Verification items for the finished model (mm, model axes). A direction names the side the tool comes from. Round coordinates to 2 decimals unless told otherwise and drop trailing zeros. Write each loop counter-clockwise with the first axis right and the second up, starting at its lowest first coordinate (ties: lowest second). Pieces come first, ordered by that corner, then holes. Notation, with made-up numbers: M -16,57.25 L -10,57.25 A20 cw -10,65.25 Z; hole C 63.5,-26 d8. An arc over 180 degrees is marked long. Use a Markdown table: item, result. Add a question column.
from build123d import *

# Parameters (mm, degrees)
FILLET_1_R      = 5
FILLET_2_R      = 10
SKETCH_2_R      = 45
SKETCH_2_R_2    = 35
EXTRUDE_1_DEPTH = 32
SKETCH_3_R      = 35
EXTRUDE_2_DEPTH = 66
SKETCH_4_R      = 37.5
EXTRUDE_3_DEPTH = 54
SKETCH_5_R      = 45
EXTRUDE_4_DEPTH = 10
SKETCH_6_R      = 37.5
EXTRUDE_5_DEPTH = 54
SKETCH_7_R      = 25
EXTRUDE_6_DEPTH = 47
SKETCH_8_R      = 20
EXTRUDE_7_DEPTH = 146
SKETCH_9_R      = 31
EXTRUDE_8_DEPTH = 3.5
SKETCH_10_R     = 32.5
EXTRUDE_9_DEPTH = 9.5


with BuildPart() as part:
    # Sketch 1 → Revolve 1 (revolve)
    with BuildSketch(Plane.XY, mode=Mode.PRIVATE) as revolve_1_sk:
        Polygon((10, 100), (50, 100), (50, 55), (40, 55), (40, 35), (0, 35), (0, 70), (10, 70), align=None)
    revolve(revolve_1_sk.sketch.rotate(Axis((-1000, 0, 0), (1, 0, 0)), 90), axis=Axis((-1000, 0, 0), (1, 0, 0)))

    # Fillet 1
    fillet_1_edges = [part.edges().sort_by_distance(p)[0] for p in [
        (10, 0, -70),
        (50, 0, -100),
        (10, 0, -100),
    ]]
    fillet(fillet_1_edges, radius=FILLET_1_R)

    # Fillet 2
    fillet_2_edges = [part.edges().sort_by_distance(p)[0] for p in [
        (40, 0, -55),
    ]]
    fillet(fillet_2_edges, radius=FILLET_2_R - 0.0001)  # a hair under: the kernel refuses the full size



with BuildPart() as body_2:
    # Sketch 2 → Extrude 1 (new body)
    with BuildSketch(Plane.ZY):
        Circle(SKETCH_2_R)
        Circle(SKETCH_2_R_2, mode=Mode.SUBTRACT)
    extrude(amount=EXTRUDE_1_DEPTH)


with BuildPart() as part_1:
    add(part.part)

    add(body_2.part)  # Extrude 2 merges body 2
    # Sketch 3 → Extrude 2 (add)
    with BuildSketch(Plane.ZY.offset(32)):
        Circle(SKETCH_3_R)
    extrude(amount=-EXTRUDE_2_DEPTH)

    # Sketch 4 → Extrude 3 (add)
    with BuildSketch(Plane.ZY.offset(32)):
        Circle(SKETCH_4_R)
    extrude(amount=EXTRUDE_3_DEPTH)

    # Sketch 5 → Extrude 4 (add)
    with BuildSketch(Plane.ZY.offset(86)):
        with Locations(Location((0, 0, 0), (0, 0, 180))):
            Circle(SKETCH_5_R)
    extrude(amount=EXTRUDE_4_DEPTH)

    # Sketch 6 → Extrude 5 (add)
    with BuildSketch(Plane.ZY.offset(96)):
        Circle(SKETCH_6_R)
    extrude(amount=EXTRUDE_5_DEPTH)

    # Sketch 7 → Extrude 6 (add)
    with BuildSketch(Plane.ZY.offset(150)):
        Circle(SKETCH_7_R)
    extrude(amount=EXTRUDE_6_DEPTH)

    # Sketch 8 → Extrude 7 (add)
    with BuildSketch(Plane.ZY.offset(197)):
        Circle(SKETCH_8_R)
    extrude(amount=EXTRUDE_7_DEPTH)

    # Sketch 9 → Extrude 8 (add)
    with BuildSketch(Plane(origin=(34, 0, 0), x_dir=(0, 0, -1), z_dir=(1, 0, 0))):
        with Locations(Location((0, 0, 0), (0, 0, 180))):
            Circle(SKETCH_9_R)
    extrude(amount=EXTRUDE_8_DEPTH)

    # Sketch 10 → Extrude 9 (add)
    with BuildSketch(Plane(origin=(37.5, 0, 0), x_dir=(0, 0, -1), z_dir=(1, 0, 0))):
        Circle(SKETCH_10_R)
    extrude(amount=EXTRUDE_9_DEPTH)


solid = part_1.part
1. Release check for a two-part mould opening along Y. For faces 4 (the cylindrical face through (2.535, 68.335, -15.175)), 5 (the cylindrical face through (37, -21, -28)), 6 (the flat face through (50, 41, 41)) record: +Y half, -Y half, draft (parallel to the pull), parting line (faces both ways), or undercut.
2. Cross-section at A-A on x = -270.5. Enter the section's corners in (y, z), plus the area to 3 significant figures.
3. Scan lines: line 1 along Y through (x, z) = (35.35, 0); line 2 along Y through (x, z) = (37.6, 0); line 3 along X through (y, z) = (24.5, 20). Record each from-to range of solid material in increasing order. Write a range as from..to.
4. Access from +Z, -Z, +X, -X, +Y, -Y to the whole of each face (thin tool, end or side, straight path). Record for faces 1 (the cylindrical face through (30.21, -30.04, 95.38)), 2 (the cylindrical face through (-90.93, 39.923, -20.765)), 3 (the cylindrical face through (35.726, -30.736, -4.036)).
5. Depth check by flat-ended pin: pin 1 Ø1.5 at (x, y) = (-253, 7.5) entering from -Z; pin 2 Ø1 at (x, y) = (-208.5, -4) entering from -Z; pin 3 Ø8 at (x, y) = (1.5, -42) entering from -Z. Enter the tip coordinate at first touch or a pass-through.
Answer:
| question | item | result |
|---|---|---|
| 1 | face 4 | parting line |
| 1 | face 5 | undercut |
| 1 | face 6 | draft |
| 2 | outline | C 0,0 d40 |
| 2 | area | 1,260 mm^2 |
| 3 | line 1 | y = -100..-35, -31..31, 35..100 |
| 3 | line 2 | y = -100..-35, -32.5..32.5, 35..100 |
| 3 | line 3 | x = -150..34, 37.5..47 |
| 4 | face 1 | +X, -X |
| 4 | face 2 | -X |
| 4 | face 3 | none |
| 5 | pin 1 | stops at z = -18.83 |
| 5 | pin 2 | stops at z = -19.69 |
| 5 | pin 3 | stops at z = -58.79 |
